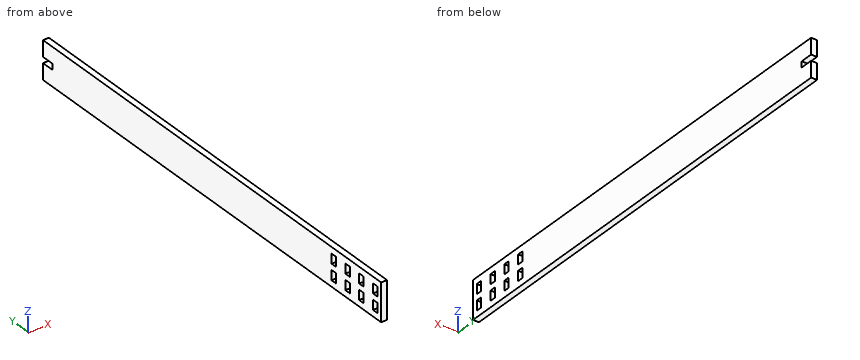
```python
from build123d import *

# Parameters (mm, degrees)
SKETCH1_W           = 228.6
SKETCH1_H           = 19.05
BOSS_EXTRUDE1_DEPTH = 2.9718
SKETCH3_W           = 6.35
SKETCH3_H           = 2.9718
CUT_EXTRUDE1_DEPTH  = 115.734681854
SKETCH4_W           = 2.9718
SKETCH4_H           = 4.8641
SKETCH4_H_2         = 4.944612775
CUT_EXTRUDE2_DEPTH  = 115.734681854


with BuildPart() as part:
    # Sketch1 → Boss-Extrude1 (new body)
    with BuildSketch(Plane.YZ):
        Rectangle(SKETCH1_W, SKETCH1_H)
    extrude(amount=BOSS_EXTRUDE1_DEPTH)

    # Sketch3 → Cut-Extrude1 (cut, through all)
    with BuildSketch(Plane.YZ.offset(2.9718)):
        with Locations((111.125, 0)):
            Rectangle(SKETCH3_W, SKETCH3_H)
    extrude(amount=-CUT_EXTRUDE1_DEPTH, mode=Mode.SUBTRACT)

    # Sketch4 → Cut-Extrude2 (cut, through all)
    with BuildSketch(Plane.YZ.offset(2.9718)):
        with Locations((-100.9523, 3.91795)):
            Rectangle(SKETCH4_W, SKETCH4_H)
        with Locations((-110.2741, 3.91795)):
            Rectangle(SKETCH4_W, SKETCH4_H)
        with Locations((-110.2741, -3.958206388)):
            Rectangle(SKETCH4_W, SKETCH4_H_2)
        with Locations((-100.9523, -3.958206388)):
            Rectangle(SKETCH4_W, SKETCH4_H_2)
        with Locations((-91.6305, 3.91795)):
            Rectangle(SKETCH4_W, SKETCH4_H)
        with Locations((-91.6305, -3.958206388)):
            Rectangle(SKETCH4_W, SKETCH4_H_2)
        with Locations((-82.3087, 3.91795)):
            Rectangle(SKETCH4_W, SKETCH4_H)
        with Locations((-82.3087, -3.958206388)):
            Rectangle(SKETCH4_W, SKETCH4_H_2)
    extrude(amount=-CUT_EXTRUDE2_DEPTH, mode=Mode.SUBTRACT)


solid = part.part
```
Check sheet for the modelled part. Datum: model origin and axes. Units: mm. Round coordinates to 2 decimals unless told otherwise and drop trailing zeros. Write item = value, one per line.
Q1. Section check A-A (x = 1.35). State how many separate pieces and enclosed holes the cut face has, and give its area (3 significant figures).
Computed:
separate_pieces = 1
enclosed_holes = 8
area = 4,220 mm^2
Q2. Go/stop test with flat-tipped pins: pin 1 (2 mm diameter, centred on y = 71, z = -1, fed in from -X); pin 2 (0.9 mm diameter, centred on x = 1, z = 0.5, fed in from +Y). Record where each tip stops, or that it passes through.
Computed:
pin_1 = 0
pin_2 = 107.95
Q3. Thickness scan on line 1 along Y through (x, z) = (1.85, 2); line 2 along Z through (x, y) = (0.5, -101.5) (3 decimals); line 3 along Y through (x, z) = (1.75, 1). Record the ranges inside material, lowest first.
Computed:
line_1 = -114.3 to -111.76, -108.79 to -102.44, -99.47 to -93.12, -90.14 to -83.79, -80.82 to 114.3
line_2 = -9.525 to -6.431, -1.486 to 1.486, 6.35 to 9.525
line_3 = -114.3 to 107.95
